Geometry: final body of the model. Coordinates: model frame, mm. A direction names the side the tool comes from. Coordinates: 2 decimals unless noted, no trailing zeros. Write each loop counter-clockwise with the first axis right and the second up, starting at its lowest first coordinate (ties: lowest second). Pieces come first, ordered by that corner, then holes.
from build123d import *

# Parameters (mm, degrees)
BOSS_EXTRUDE1_DEPTH = 20
BOSS_EXTRUDE4_DEPTH = 2
SKETCH9_R           = 2.1
BOSS_EXTRUDE5_DEPTH = 4


with BuildPart() as part:
    # Sketch1 → Boss-Extrude1 (new body)
    with BuildSketch(Plane(origin=(0, 0, 0), x_dir=(1, 0, 0), z_dir=(0, 1, 0))):
        with BuildLine():
            Line((-47.421696664, 8.493167766), (-32.921696664, 8.493167766))
            ThreePointArc((-32.921696664, 8.493167766), (-28.309146849, 7.256965456), (-24.933036081, 3.879734634))
            Line((-24.933036081, 3.879734634), (-17.636401145, -8.844865692))
            ThreePointArc((-17.636401145, -8.844865692), (-17.820612025, -17.958509448), (-25.745395692, -22.46297834))
            Line((-25.745395692, -22.46297834), (-54.645395692, -22.46297834))
            ThreePointArc((-54.645395692, -22.46297834), (-62.607823184, -17.894709582), (-62.682753297, -8.715182552))
            Line((-62.682753297, -8.715182552), (-55.348980831, 3.984497041))
            ThreePointArc((-55.348980831, 3.984497041), (-51.981574567, 7.287152643), (-47.421696664, 8.493167766))
        make_face()
        with BuildLine():
            Line((-47.421696664, 6.493167766), (-32.921696664, 6.493167766))
            ThreePointArc((-32.921696664, 6.493167766), (-29.310446688, 5.525665157), (-26.666587696, 2.882334433))
            Line((-26.666587696, 2.882334433), (-19.384059263, -9.817665567))
            ThreePointArc((-19.384059263, -9.817665567), (-19.544805292, -16.944941641), (-25.745395692, -20.46297834))
            Line((-25.745395692, -20.46297834), (-54.645395692, -20.46297834))
            ThreePointArc((-54.645395692, -20.46297834), (-60.878636724, -16.889747838), (-60.944972269, -9.705259715))
            Line((-60.944972269, -9.705259715), (-53.623842396, 2.97252707))
            ThreePointArc((-53.623842396, 2.97252707), (-50.987559904, 5.551646576), (-47.421696664, 6.493167766))
        make_face(mode=Mode.SUBTRACT)
    extrude(amount=BOSS_EXTRUDE1_DEPTH)

    # Sketch8 → Boss-Extrude4 (add)
    with BuildSketch(Plane(origin=(0, 20, 0), x_dir=(1, 0, 0), z_dir=(0, 1, 0))):
        with BuildLine():
            Line((-55.348980831, 3.984497041), (-62.682753297, -8.715182552))
            ThreePointArc((-62.682753297, -8.715182552), (-62.607823184, -17.894709582), (-54.645395692, -22.462978339))
            Line((-54.645395692, -22.462978339), (-25.745395692, -22.46297834))
            ThreePointArc((-25.745395692, -22.46297834), (-17.820612025, -17.958509448), (-17.636401145, -8.844865692))
            Line((-17.636401145, -8.844865692), (-24.933036081, 3.879734634))
            ThreePointArc((-24.933036081, 3.879734634), (-28.309146849, 7.256965456), (-32.921696664, 8.493167766))
            Line((-32.921696664, 8.493167766), (-47.421696664, 8.493167766))
            ThreePointArc((-47.421696664, 8.493167766), (-51.981574567, 7.287152643), (-55.348980831, 3.984497041))
        make_face()
    extrude(amount=BOSS_EXTRUDE4_DEPTH)

    # Sketch9 → Boss-Extrude5 (add)
    # profile 1 of 2: a face of its own
    with BuildSketch(Plane(origin=(0, 22, 0), x_dir=(1, 0, 0), z_dir=(0, 1, 0))):
        with BuildLine():
            Line((-59.674100701, 4.493496912), (-56.210189139, 2.493167766))
            Line((-56.210189139, 2.493167766), (-61.211012004, -6.166611138))
            Line((-61.211012004, -6.166611138), (-64.674923565, -4.166281993))
            ThreePointArc((-64.674923565, -4.166281993), (-66.504401585, 2.664018892), (-59.674100701, 4.493496912))
        make_face()
        with Locations(Location((-62.174512133, 0.16360746, 0), (0, 0, 270))):
            Circle(SKETCH9_R, mode=Mode.SUBTRACT)
    # profile 2 of 2: a face of its own
    with BuildSketch(Plane(origin=(0, 22, 0), x_dir=(1, 0, 0), z_dir=(0, 1, 0))):
        with BuildLine():
            Line((-19.154852081, -6.198807979), (-24.142409797, 2.468617708))
            Line((-24.142409797, 2.468617708), (-20.675439522, 4.463640794))
            ThreePointArc((-20.675439522, 4.463640794), (-13.847947821, 2.623706808), (-15.687881807, -4.203784893))
            Line((-15.687881807, -4.203784893), (-19.154852081, -6.198807979))
        make_face()
        with Locations(Location((-18.181660664, 0.12992795, 0), (0, 0, 90))):
            Circle(SKETCH9_R, mode=Mode.SUBTRACT)
    extrude(amount=-BOSS_EXTRUDE5_DEPTH)


solid = part.part
Item 1: Set-up query: faces 1 (the flat face through (-16, 18, -1)), 2 (the flat face through (-60, 18, -2)), 3 (the cylindrical face through (-19.49, 9.86, 16.85)), 4 (the flat face through (-22.426, 20.028, -3.456)). Return all of +Z, -Z, +X, -X, +Y, -Y with unobstructed straight access to the full face (end or side cutting, diameter ignored); none if empty.
Derived:
face 1: -Z, +X, -Y
face 2: -Z, -X, -Y
face 3: -Y
face 4: -Z, +Y, -Y
Item 2: Pull-direction query (X, two-part tool) for faces 5 (the flat face through (-17.4, 20.03, 5.19)), 6 (the flat face through (-40, 11, -8.493)), 7 (the cylindrical face through (-19.95, 20.03, -1.26)); classes: released by +X, released by -X, zero draft, split by the parting line, or undercut.
Derived:
face 5: released by +X
face 6: zero draft
face 7: undercut
Item 3: Section D-D, the plane y = 19. Output: boundary loops of the cut face in (x, z).
Derived:
outline: (-64.67, 4.17) arc R5 ccw to (-59.67, -4.49) - (-56.21, -2.49) - (-55.35, -3.98) arc R9.22 ccw to (-47.42, -8.49) - (-32.92, -8.49) arc R9.22 ccw to (-24.93, -3.88) - (-24.13, -2.48) - (-20.68, -4.46) arc R5 ccw to (-15.69, 4.2) - (-19.15, 6.2) - (-17.64, 8.84) arc R9.22 ccw to (-25.75, 22.46) - (-54.65, 22.46) arc R9.22 ccw to (-62.68, 8.72) - (-61.21, 6.17) - close; hole circle Ø4.2 at (-62.17, -0.16); hole (-60.94, 9.71) - (-53.62, -2.97) arc R7.22 ccw to (-47.42, -6.49) - (-32.92, -6.49) arc R7.22 ccw to (-26.67, -2.88) - (-19.38, 9.82) arc R7.22 ccw to (-25.75, 20.46) - (-54.65, 20.46) arc R7.22 ccw to start; hole circle Ø4.2 at (-18.18, -0.13)
Item 4: Section C-C, the plane z = 1. Output: boundary loops of the cut face in (x, y).
Derived:
outline: (-67.04, 18) - (-63.92, 18) - (-63.92, 22) - (-67.04, 22) - close; (-60.43, 18) - (-58.23, 18) - (-58.23, 0) - (-55.92, 0) - (-55.92, 20) - (-24.44, 20) - (-24.44, 0) - (-22.13, 0) - (-22.13, 18) - (-19.95, 18) - (-19.95, 22) - (-60.43, 22) - close; (-16.41, 18) - (-13.31, 18) - (-13.31, 22) - (-16.41, 22) - close
Item 5: Section B-B, the plane x = -43.5. Output: boundary loops of the cut face in (y, z).
Derived:
outline: (0, -8.49) - (22, -8.49) - (22, 22.46) - (0, 22.46) - (0, 20.46) - (20, 20.46) - (20, -6.49) - (0, -6.49) - close
Item 6: Section A-A, the plane y = 14.75. Output: boundary loops of the cut face in (x, z), plus the area to 3 significant figures.
Derived:
outline: (-62.68, 8.72) - (-55.35, -3.98) arc R9.22 ccw to (-47.42, -8.49) - (-32.92, -8.49) arc R9.22 ccw to (-24.93, -3.88) - (-17.64, 8.84) arc R9.22 ccw to (-25.75, 22.46) - (-54.65, 22.46) arc R9.22 ccw to start; hole (-60.94, 9.71) - (-53.62, -2.97) arc R7.22 ccw to (-47.42, -6.49) - (-32.92, -6.49) arc R7.22 ccw to (-26.67, -2.88) - (-19.38, 9.82) arc R7.22 ccw to (-25.75, 20.46) - (-54.65, 20.46) arc R7.22 ccw to start
area: 248 mm2
Item 7: Pin query (flat end, axial travel): pin 1 (2 mm diameter, centred on x = -53.5, z = 2.5, fed in from -Y); pin 2 (1 mm diameter, centred on y = 8, z = -5, fed in from -X); pin 3 (1 mm diameter, centred on y = 8, z = 15, fed in from -X). Return the tip coordinate at first contact, or that it passes through.
Derived:
pin 1: stops at y = 20
pin 2: stops at x = -55.02
pin 3: stops at x = -63.78
Item 8: Material intervals for probe 1 along Z at (x, y) = (-42, 3.25); probe 2 along Y at (x, z) = (-56.5, 9); probe 3 along Z at (x, y) = (-53.5, 3.75), sorted ascending.
Derived:
probe 1: z = -8.49 to -6.49, 20.46 to 22.46
probe 2: y = 20 to 22
probe 3: z = -6.21 to -3.17, 20.46 to 22.46
